Could you check a few things on this model? Use its own coordinates, in mm. A direction names the side the tool comes from. Give positions to 0.01 mm unless a question says otherwise; leave off trailing zeros. Write each loop counter-clockwise with the first axis right and the second up, starting at its lowest first coordinate (ties: lowest second). Pieces come first, ordered by that corner, then holes. Notation, with made-up numbers: (-28, -30.75) - (24, -30.75) arc R3 ccw to (24, -26.75) - close; hole circle Ø3 at (-20, 16.5). An arc over 180 degrees is marked (long way). Answer in a Markdown table with one row per item.
from build123d import *

# Parameters (mm, degrees)
BOSS_EXTRUDE1_DEPTH      = 6.35
M5_CLEARANCE_HOLE1_D     = 5.5
M5_CLEARANCE_HOLE1_DEPTH = 18.75
M5_CLEARANCE_HOLE1_TIP   = 1.652366702
FILLET1_R                = 3.175
M5_CLEARANCE_HOLE2_D     = 5.5
M5_CLEARANCE_HOLE2_DEPTH = 18.75
M5_CLEARANCE_HOLE2_TIP   = 1.652366702


with BuildPart() as part:
    # Sketch1 → Boss-Extrude1 (new body)
    with BuildSketch(Plane.XY):
        Polygon((38.1, 25.4), (38.1, 54.890872965), (142.990872965, 54.890872965), (142.990872965, 38.890872965), (63.5, 38.890872965), (63.5, -22.890872965), (142.990872965, -22.890872965), (142.990872965, -38.890872965), (38.1, -38.890872965), (38.1, -25.4), (-38.1, -25.4), (-38.1, 25.4), align=None)
    extrude(amount=BOSS_EXTRUDE1_DEPTH)

    # M5 Clearance Hole1
    with Locations(Plane.XY.offset(6.35)):
        with Locations((134.990872965, 46.890872965), (134.990872965, -30.890872965), (57.209127035, 46.890872965), (57.209127035, -30.890872965)):
            Hole(M5_CLEARANCE_HOLE1_D / 2, depth=M5_CLEARANCE_HOLE1_DEPTH)
            with Locations((0, 0, -(M5_CLEARANCE_HOLE1_DEPTH + M5_CLEARANCE_HOLE1_TIP / 2))):  # 118° drill point
                Cone(0, M5_CLEARANCE_HOLE1_D / 2, M5_CLEARANCE_HOLE1_TIP, mode=Mode.SUBTRACT)

    # Fillet1
    fillet1_edges = [part.edges().sort_by_distance(p)[0] for p in [
        (38.1, 25.4, 3.175),
        (63.5, 38.890872965, 3.175),
        (63.5, -22.890872965, 3.175),
        (38.1, -25.4, 3.175),
    ]]
    fillet(fillet1_edges, radius=FILLET1_R)

    # M5 Clearance Hole2
    with Locations(Plane.XY.offset(6.35)):
        with Locations((-25.4, 12.7), (25.4, 12.7), (25.4, -12.7), (-25.4, -12.7)):
            Hole(M5_CLEARANCE_HOLE2_D / 2, depth=M5_CLEARANCE_HOLE2_DEPTH)
            with Locations((0, 0, -(M5_CLEARANCE_HOLE2_DEPTH + M5_CLEARANCE_HOLE2_TIP / 2))):  # 118° drill point
                Cone(0, M5_CLEARANCE_HOLE2_D / 2, M5_CLEARANCE_HOLE2_TIP, mode=Mode.SUBTRACT)


solid = part.part
1) Imagine slicing it at B-B (x = 25.4). List the corners of the cut face in (y, z) for me.
Check values:
| item | result |
|---|---|
| outline | (-25.4, 0) - (-15.45, 0) - (-15.45, 6.35) - (-25.4, 6.35) - close; (-9.95, 0) - (9.95, 0) - (9.95, 6.35) - (-9.95, 6.35) - close; (15.45, 0) - (25.4, 0) - (25.4, 6.35) - (15.45, 6.35) - close |
2) Imagine slicing it at D-D (z = 4.75). State how many separate pieces and enclosed holes the cut face has, then the cut area to 3 significant figures.
Check values:
| item | result |
|---|---|
| separate pieces | 1 |
| enclosed holes | 8 |
| area | 8,620 mm2 |
3) We'd pull the mould along X, two halves only. Please class faces 1 (the face through (105, 38.891, 3)), 2 (the face through (37.15, -26.31, 3.22)), 3 (the face through (24.13, -15.14, 3.13)), 4 (the face through (137.173, -32.564, 3.131)): +X half, -X half, draft (parallel to the pull), parting line (faces both ways), or undercut.
Check values:
| item | result |
|---|---|
| face 1 | draft |
| face 2 | -X half |
| face 3 | undercut |
| face 4 | undercut |
4) Will these pins go through, and if not, where does the flat tip stop? P1, Ø1.9, axis at y = -1.5, z = 1.5, coming from the +X side; P2, Ø7, axis at x = 25.4, y = 12.7, coming from the +Z side; P3, Ø4.5, axis at x = -25.4, y = 12.7, coming from the -Z side; P4, Ø3, axis at x = -9.5, z = 1.5, coming from the +Y side.
Check values:
| item | result |
|---|---|
| P1 | stops at x = 63.5 |
| P2 | stops at z = 6.35 |
| P3 | passes through |
| P4 | stops at y = 25.4 |
5) If I drill on line 1 (Y direction, x = 25.4, z = 5); line 2 (Y direction, x = 105, z = 4); line 3 (X direction, y = 13.5, z = 2.25), over which ranges is the centre line in solid material (lowest first)?
Check values:
| item | result |
|---|---|
| line 1 | y = -25.4 to -15.45, -9.95 to 9.95, 15.45 to 25.4 |
| line 2 | y = -38.89 to -22.89, 38.89 to 54.89 |
| line 3 | x = -38.1 to -28.03, -22.77 to 22.77, 28.03 to 63.5 |
6) Imagine slicing it at C-C (y = -12.7). List the corners of the cut face in (x, z) for me, then the cut area to 3 significant figures.
Check values:
| item | result |
|---|---|
| outline | (-38.1, 0) - (-28.15, 0) - (-28.15, 6.35) - (-38.1, 6.35) - close; (-22.65, 0) - (22.65, 0) - (22.65, 6.35) - (-22.65, 6.35) - close; (28.15, 0) - (63.5, 0) - (63.5, 6.35) - (28.15, 6.35) - close |
| area | 575 mm2 |
7) On a 3-axis mill with a long thin cutter (end or side, diameter ignored), from which of +Z, -Z, +X, -X, +Y, -Y can I reach the whole of each face in a straight line? I mean faces 5 (the face through (38.1, -34, 3)), 6 (the face through (-2, 25.4, 3)), 7 (the face through (64.455, 37.985, 3.219)). Say none if no direction works.
Check values:
| item | result |
|---|---|
| face 5 | +Z, -Z, -X, -Y |
| face 6 | +Z, -Z, -X, +Y |
| face 7 | +Z, -Z, +X |
8) Imagine slicing it at A-A (x = 119). List the corners of the cut face in (y, z) for me.
Check values:
| item | result |
|---|---|
| outline | (-38.89, 0) - (-22.89, 0) - (-22.89, 6.35) - (-38.89, 6.35) - close; (38.89, 0) - (54.89, 0) - (54.89, 6.35) - (38.89, 6.35) - close |
